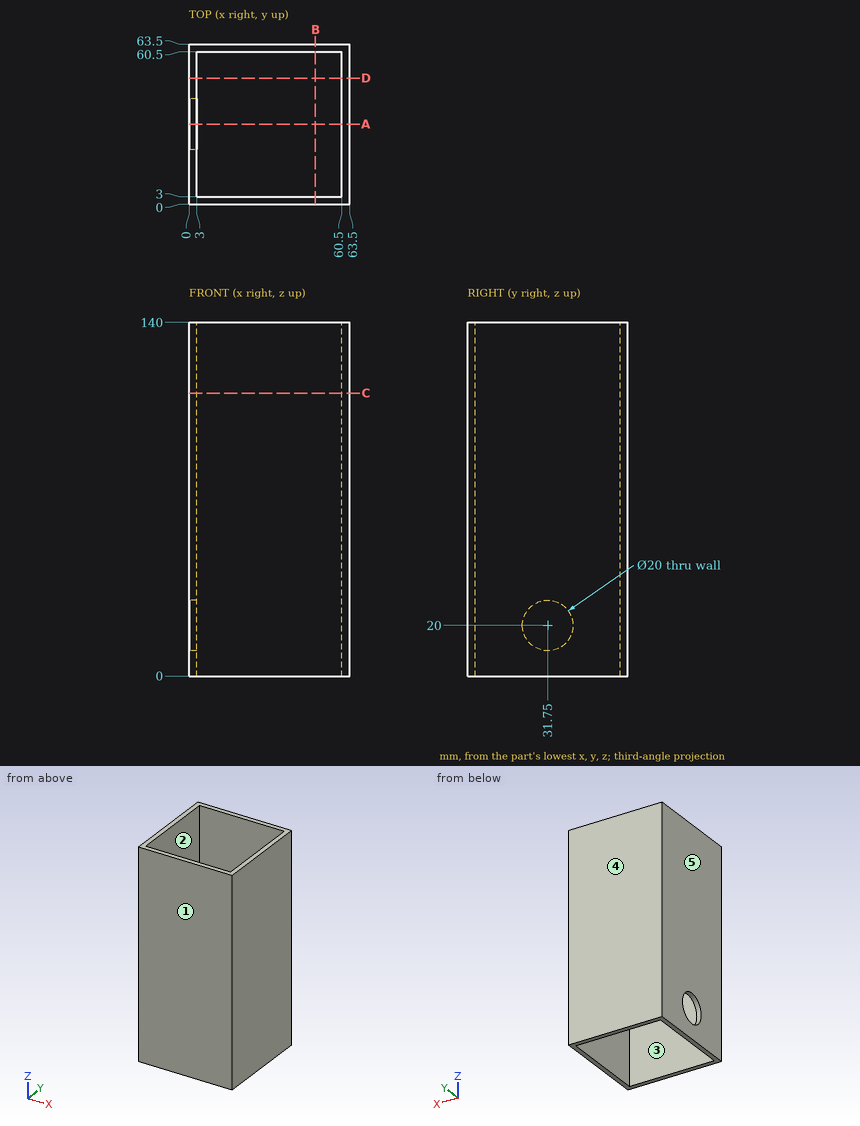
Could you check a few things on this drawing? It's one solid part, dimensions in mm from its lowest x, y, z. A direction names the side the tool comes from. Coordinates: 2 decimals unless noted, no trailing zeros. Write each loop counter-clockwise with the first axis right and the second up, starting at its lowest first coordinate (ties: lowest second). Pieces come first, ordered by that corner, then holes. Notation, with made-up numbers: (43.5, 87.5) - (92.5, 87.5) arc R19 ccw to (92.5, 102.5) - close; hole circle Ø8 at (74.25, 23). An arc over 180 degrees is marked (long way). Put each result on its own line as item: value. Start each with the question number.
Q1. I want a section at B-B on x = 50. Write out the boundary of the cut face in (y, z).
Q2. I want a section at C-C on z = 112. Write out the boundary of the cut face in (x, y).
Q3. I want a section at A-A on y = 31.75. Write out the boundary of the cut face in (x, z), plus the area to 3 significant figures.
Q4. Thinking about a two-plate mould opening in Y: for the marked faces 3, 4 and 5, which applies, pulls with the +Y half, pulls with the -Y half, needs draft (parallel to the pull), parting line crosses it, or undercut?
Q5. Which directions (+Z, -Z, +X, -X, +Y, -Y) give clear straight access to the entire face, cutting with the end or side of a thin tool? Please do the marked faces 1 and 2.
Q6. Please list where these lines run through material, in increasing order: L1, parallel to X at y = 30.5, z = 65.5; L2, parallel to Z at x = 0.9, y = 31.75.
Q7. I'm going to push flat-ended pins straight in: P1, Ø10, axis at y = 39.5, z = 59.5, coming from the -X side; P2, Ø16, axis at y = 31.75, z = 20, coming from the -X side. Where does each tip first touch, or does it pass through?
Checks:
1. outline: (0, 0) - (3, 0) - (3, 140) - (0, 140) - close; (60.5, 0) - (63.5, 0) - (63.5, 140) - (60.5, 140) - close
2. outline: (0, 0) - (63.5, 0) - (63.5, 63.5) - (0, 63.5) - close; hole (3, 3) - (60.5, 3) - (60.5, 60.5) - (3, 60.5) - close
3. outline: (0, 0) - (3, 0) - (3, 10) - (0, 10) - close; (0, 30) - (3, 30) - (3, 140) - (0, 140) - close; (60.5, 0) - (63.5, 0) - (63.5, 140) - (60.5, 140) - close
3. area: 780 mm²
4. face 3: undercut
4. face 4: pulls with the +Y half
4. face 5: needs draft
5. face 1: +Z, -Z, +X, -X, -Y
5. face 2: +Z, -Z
6. L1: 0 to 3, 60.5 to 63.5
6. L2: 0 to 10, 30 to 140
7. P1: x = 0
7. P2: x = 60.5
